For this review, use the dimensioned drawing (mm, ordinates from the lowest corner) and the shaded views. Give positions to 0.01 mm unless a question says otherwise; leave off trailing zeros. Write each loop counter-clockwise with the first axis right and the second up, starting at its lowest first coordinate (ties: lowest second). Pieces come first, ordered by that corner, then holes. Notation, with made-up numbers: M 89.5,6 L 103.5,6 A25 ccw 103.5,31 Z; hole C 71.25,1 d5. An arc over 180 degrees is marked long. Use a Markdown table: item, result. Add a question column.
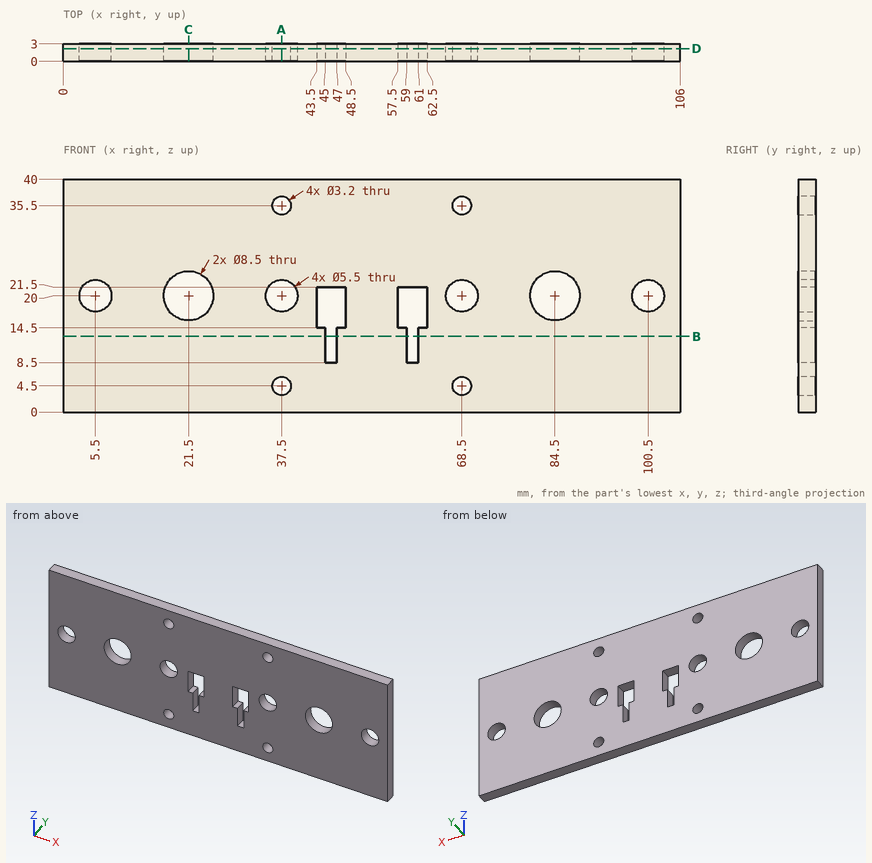
(1) Add section A-A on x = 37.5. Give the boundary of the cut face in (y, z), then the cut area to 3 significant figures.
(2) Add section D-D on y = 2.2. Give the number of separate pieces and of enclosed holes in the cut face, then the cut area to 3 significant figures.
(3) Add section B-B on z = 13. Give the boundary of the cut face in (x, y).
(4) Add section C-C on x = 21.5. Give the boundary of the cut face in (y, z), then the cut area to 3 significant figures.
(5) For pin 1 (5 mm diameter, centred on x = 84.5, z = 20, fed in from +Y), flat-tipped, find the tip position at first contact; note if it passes through.
(6) Wall thickness on L1, parallel to X at y = 2.9, z = 35.5; L2, parallel to Z at x = 68.5, y = 1; L3, parallel to X at y = 2.4, z = 5.5: over which ranges is each line inside the solid? List them lowest first.
From the geometry:
| question | item | result |
|---|---|---|
| 1 | outline | M 0,0 L 3,0 L 3,2.9 L 0,2.9 Z; M 0,6.1 L 3,6.1 L 3,17.25 L 0,17.25 Z; M 0,22.75 L 3,22.75 L 3,33.9 L 0,33.9 Z; M 0,37.1 L 3,37.1 L 3,40 L 0,40 Z |
| 1 | area | 84.3 mm^2 |
| 2 | separate pieces | 1 |
| 2 | enclosed holes | 12 |
| 2 | area | 3,910 mm^2 |
| 3 | outline | M 0,0 L 45,0 L 45,3 L 0,3 Z; M 47,0 L 59,0 L 59,3 L 47,3 Z; M 61,0 L 106,0 L 106,3 L 61,3 Z |
| 4 | outline | M 0,0 L 3,0 L 3,15.75 L 0,15.75 Z; M 0,24.25 L 3,24.25 L 3,40 L 0,40 Z |
| 4 | area | 94.5 mm^2 |
| 5 | pin 1 | passes through |
| 6 | L1 | x = 0 to 35.9, 39.1 to 66.9, 70.1 to 106 |
| 6 | L2 | z = 0 to 2.9, 6.1 to 17.25, 22.75 to 33.9, 37.1 to 40 |
| 6 | L3 | x = 0 to 36.25, 38.75 to 67.25, 69.75 to 106 |
